Work out the finished part from the listing and answer in its coordinate system (mm). A direction names the side the tool comes from. Coordinates: 2 decimals unless noted, no trailing zeros. Write each loop counter-clockwise with the first axis right and the second up, starting at its lowest first coordinate (ties: lowest second). Pieces come first, ordered by that corner, then holes. Notation, with made-up numbers: M 62.25,65.5 L 97.25,65.5 A24 ccw 97.25,92.5 Z; hole C -21,-10.75 d4. An arc over 180 degrees is marked long. Use CSV: the item, a comma, the result in double quotes.
from build123d import *

# Parameters (mm, degrees)
EXTRUDE_1_DEPTH     = 17
SKETCH_2_R          = 3
CUT_EXTRUDE_1_DEPTH = 10
CUT_EXTRUDE_2_DEPTH = 4
SKETCH_5_R          = 2.7
CUT_EXTRUDE_3_DEPTH = 20


with BuildPart() as part:
    # 草图1 → 凸台-拉伸1 (new body)
    with BuildSketch(Plane.XY):
        with BuildLine():
            Line((-57.689289948, -69), (57.689289948, -69))
            ThreePointArc((57.689289948, -69), (69.131727984, -69.131727984), (69, -57.689289948))
            Line((69, -57.689289948), (69, 57.689289948))
            ThreePointArc((69, 57.689289948), (71.327983317, 65.000871727), (66.431261108, 70.908565529))
            Line((66.431261108, 70.908565529), (27.260903157, 86.486659817))
            ThreePointArc((27.260903157, 86.486659817), (26.344978295, 87.222183323), (26, 88.345082765))
            Line((26, 88.345082765), (26, 95.5))
            ThreePointArc((26, 95.5), (25.414213562, 96.914213562), (24, 97.5))
            Line((24, 97.5), (-24, 97.5))
            ThreePointArc((-24, 97.5), (-25.414213562, 96.914213562), (-26, 95.5))
            Line((-26, 95.5), (-26, 88.345082765))
            ThreePointArc((-26, 88.345082765), (-26.344978295, 87.222183323), (-27.260903157, 86.486659817))
            Line((-27.260903157, 86.486659817), (-66.431261108, 70.908565529))
            ThreePointArc((-66.431261108, 70.908565529), (-71.327983317, 65.000871727), (-69, 57.689289948))
            Line((-69, 57.689289948), (-69, -57.689289948))
            ThreePointArc((-69, -57.689289948), (-69.131727984, -69.131727984), (-57.689289948, -69))
        make_face()
    extrude(amount=EXTRUDE_1_DEPTH)

    # 草图2 → 切除-拉伸1 (cut)
    with BuildSketch(Plane.XY.offset(17)):
        with Locations((-63.474873734, 63.474873734)):
            Circle(SKETCH_2_R)
        with Locations((63.474873734, 63.474873734)):
            Circle(SKETCH_2_R)
        with Locations((-63.474873734, -63.474873734)):
            Circle(SKETCH_2_R)
        with Locations((63.474873734, -63.474873734)):
            Circle(SKETCH_2_R)
    extrude(amount=-CUT_EXTRUDE_1_DEPTH, mode=Mode.SUBTRACT)

    # 草图3 → 切除-拉伸2 (cut)
    with BuildSketch(Plane.XY.offset(17)):
        with BuildLine():
            Line((-20.708333333, 77.408885729), (-5.833333333, 84.2268308))
            ThreePointArc((-5.833333333, 84.2268308), (-2.985328189, 85.178004811), (0, 85.5))
            ThreePointArc((0, 85.5), (2.985328189, 85.178004811), (5.833333333, 84.2268308))
            Line((5.833333333, 84.2268308), (20.708333333, 77.408885729))
            ThreePointArc((20.708333333, 77.408885729), (24.5, 71.5), (20.708333333, 65.591114271))
            Line((20.708333333, 65.591114271), (5.833333333, 58.7731692))
            ThreePointArc((5.833333333, 58.7731692), (2.985328189, 57.821995189), (0, 57.5))
            ThreePointArc((0, 57.5), (-2.985328189, 57.821995189), (-5.833333333, 58.7731692))
            Line((-5.833333333, 58.7731692), (-20.708333333, 65.591114271))
            ThreePointArc((-20.708333333, 65.591114271), (-24.5, 71.5), (-20.708333333, 77.408885729))
        make_face()
    extrude(amount=-CUT_EXTRUDE_2_DEPTH, mode=Mode.SUBTRACT)

    # 草图5 → 切除-拉伸3 (cut)
    with BuildSketch(Plane.XY.offset(13)):
        with Locations((-18, 71.5)):
            Circle(SKETCH_5_R)
        with Locations((18, 71.5)):
            Circle(SKETCH_5_R)
    extrude(amount=-CUT_EXTRUDE_3_DEPTH, mode=Mode.SUBTRACT)


solid = part.part
Item 1: The part is cut by section C-C (y = 7.5). Write down the section's boundary in (x, z).
Answer:
outline,"M -69,0 L 69,0 L 69,17 L -69,17 Z"
Item 2: A tool of negligible diameter and unlimited length cuts with its end or side. For faces 4 (the face through (69, -1, 8)), 5 (the face through (-63.87, -60.5, 12.07)), 6 (the face through (-71.306, 65.111, 8.381)), 7 (the face through (17.415, 68.864, 6.591)), 8 (the face through (26, 92, 8)), from which of +Z, -Z, +X, -X, +Y, -Y can it reach the whole face along a straight path? Write none if from no direction.
Answer:
face 4,"+Z, -Z, +X"
face 5,"+Z"
face 6,"+Z, -Z, -X"
face 7,"+Z, -Z"
face 8,"+Z, -Z, +X, +Y"
Item 3: The part is cut by section A-A (z = 2.75). Write down the section's boundary in (x, y), then the cut area to 3 significant figures.
Answer:
outline,"M -69,-57.69 A8 ccw long -57.69,-69 L 57.69,-69 A8 ccw long 69,-57.69 L 69,57.69 A8 ccw 66.43,70.91 L 27.26,86.49 A2 cw 26,88.35 L 26,95.5 A2 ccw 24,97.5 L -24,97.5 A2 ccw -26,95.5 L -26,88.35 A2 cw -27.26,86.49 L -66.43,70.91 A8 ccw -69,57.69 Z; hole C -18,71.5 d5.4; hole C 18,71.5 d5.4"
area,"21,400 mm2"
Item 4: Given pin 1 (3.5 mm diameter, centred on x = 63.47, y = 63.47, fed in from +Z); pin 2 (1.5 mm diameter, centred on x = 37, z = 14, fed in from +Y); pin 3 (2 mm diameter, centred on x = 20.5, z = 12.5, fed in from -Y), each flat-ended and moving along its own axis, determine where each tip first touches the part or whether it passes through.
Answer:
pin 1,"stops at z = 7"
pin 2,"stops at y = 82.91"
pin 3,"stops at y = -69"
Item 5: Consider probe 1 along Y at (x, z) = (-18, 9); probe 2 along X at (y, z) = (41, 11.5); probe 3 along X at (y, z) = (88, 15). Determine where each line is inside the solid, lowest interval first.
Answer:
probe 1,"y = -69 to 68.8, 74.2 to 97.5"
probe 2,"x = -69 to 69"
probe 3,"x = -26.03 to 26.03"
Item 6: The part is cut by section D-D (x = 37). Write down the section's boundary in (y, z).
Answer:
outline,"M -69,0 L 82.61,0 L 82.61,17 L -69,17 Z"
Item 7: For a pull along Y with two mould halves and no side action, classify faces 1 (the face through (-1, -69, 8)), 2 (the face through (13.167, 80.866, 15.028)), 3 (the face through (-26, 92, 8)) as released by +Y, released by -Y, zero draft, split by the parting line, or undercut.
Answer:
face 1,"released by -Y"
face 2,"undercut"
face 3,"zero draft"
Item 8: The part is cut by section B-B (x = 18). Write down the section's boundary in (y, z), then the cut area to 3 significant figures.
Answer:
outline,"M -69,0 L 68.8,0 L 68.8,13 L 64.35,13 L 64.35,17 L -69,17 Z; M 74.2,0 L 97.5,0 L 97.5,17 L 78.65,17 L 78.65,13 L 74.2,13 Z"
area,"2,700 mm2"
